Check sheet for the modelled part. Datum: model origin and axes. Units: mm. A direction names the side the tool comes from. Coordinates: 2 decimals unless noted, no trailing zeros. Write each loop counter-clockwise with the first axis right and the second up, starting at its lowest first coordinate (ties: lowest second). Pieces come first, ordered by that corner, then holes. Notation, with made-up numbers: M 22,61 L 79,61 A22 cw 79,97 Z; hole C 28,12.25 d11. An arc over 180 degrees is marked long. Answer as CSV lines item,"result". Start each with the question number.
Q1. Sectioned sample at C-C, the plane x = 1.25. Record the cut outline in (y, z).
Q2. Access from +Z, -Z, +X, -X, +Y, -Y to the whole of each face (thin tool, end or side, straight path). Record for faces 1 (the flat face through (-1.5, -7.4, 0.5)), 2 (the flat face through (1, -7, 0)), 3 (the flat face through (-1.5, -15, 0)), 4 (the flat face through (1.5, -7.4, -0.5)).
Q3. Sectioned sample at D-D, the plane x = 0. Record the cut outline in (y, z).
Q4. Depth check by flat-ended pin: pin 1 Ø1.1 at (y, z) = (-7, 0) entering from +X; pin 2 Ø0.5 at (x, y) = (-1.5, -9) entering from -Z; pin 3 Ø1.1 at (x, y) = (1.5, -7.5) entering from +Z. Enter the tip coordinate at first touch or a pass-through.
Q5. Thickness scan on line 1 along Y through (x, z) = (-1, -3); line 2 along Z through (x, y) = (-1.75, -7.25); line 3 along Z through (x, y) = (2.25, 6.5). Record the ranges inside material, lowest first. Write a range as from..to.
Q6. Mould release check, pull along X, two halves, no side actions. Record for faces 5 (the flat face through (0, 9, 0)), 6 (the flat face through (2, -7, 0)), 7 (the flat face through (-1, -7, 0)), 8 (the flat face through (-2, -7, 0)): pulls with the +X half, pulls with the -X half, needs draft (parallel to the pull), parting line crosses it, or undercut.
Q7. Sectioned sample at A-A, the plane y = -0.25. Record the cut outline in (x, z).
Q8. Sectioned sample at B-B, the plane z = 0. Record the cut outline in (x, y).
from build123d import *

# Parameters (mm, degrees)
SKETCH1_R           = 3.5
BOSS_EXTRUDE1_DEPTH = 9
SKETCH2_W           = 1
SKETCH2_H           = 1
BOSS_EXTRUDE2_DEPTH = 24


with BuildPart() as part:
    # Sketch1 → Boss-Extrude1 (new body)
    with BuildSketch(Plane(origin=(0, 0, 0), x_dir=(1, 0, 0), z_dir=(0, 1, 0))):
        Circle(SKETCH1_R)
    extrude(amount=BOSS_EXTRUDE1_DEPTH)

    # Sketch2 → Boss-Extrude2 (add)
    with BuildSketch(Plane(origin=(0, 9, 0), x_dir=(1, 0, 0), z_dir=(0, 1, 0))):
        with Locations((-1.5, 0)):
            Rectangle(SKETCH2_W, SKETCH2_H)
        with Locations((1.5, 0)):
            Rectangle(SKETCH2_W, SKETCH2_H)
    extrude(amount=-BOSS_EXTRUDE2_DEPTH)


solid = part.part
Output:
1,outline,"M -15,-0.5 L 0,-0.5 L 0,-3.27 L 9,-3.27 L 9,3.27 L 0,3.27 L 0,0.5 L -15,0.5 Z"
2,face 1,"+Z, +X, -X, -Y"
2,face 2,"+Z, -Z, -Y"
2,face 3,"+Z, -Z, +X, -X, -Y"
2,face 4,"-Z, +X, -X, -Y"
3,outline,"M 0,-3.5 L 9,-3.5 L 9,3.5 L 0,3.5 Z"
4,pin 1,"stops at x = 2"
4,pin 2,"stops at z = -0.5"
4,pin 3,"stops at z = 0.5"
5,line 1,"y = 0..9"
5,line 2,"z = -0.5..0.5"
5,line 3,"z = -2.68..2.68"
6,face 5,"needs draft"
6,face 6,"pulls with the +X half"
6,face 7,"undercut"
6,face 8,"pulls with the -X half"
7,outline,"M -2,-0.5 L -1,-0.5 L -1,0.5 L -2,0.5 Z; M 1,-0.5 L 2,-0.5 L 2,0.5 L 1,0.5 Z"
8,outline,"M -3.5,0 L -2,0 L -2,-15 L -1,-15 L -1,0 L 1,0 L 1,-15 L 2,-15 L 2,0 L 3.5,0 L 3.5,9 L -3.5,9 Z"
